Geometry: see drawing. Coordinates: mm, zero at the bounding-box minimum. Give positions to 0.01 mm unless a question says otherwise; leave off trailing zeros. Order: outer loops, then holes, each group sorted by start corner. A loop starts at its lowest first (then second) coordinate and runs counter-clockwise, first axis right, second up. Notation, with made-up numbers: (4.5, -35.5) -> (50.5, -35.5) arc R31 cw to (50.5, 1.5) -> close; hole circle Ø6 at (-11.75, 78). An arc over 180 degrees is marked (long way). Use one line per item in the form item = value. Start each with the question number.
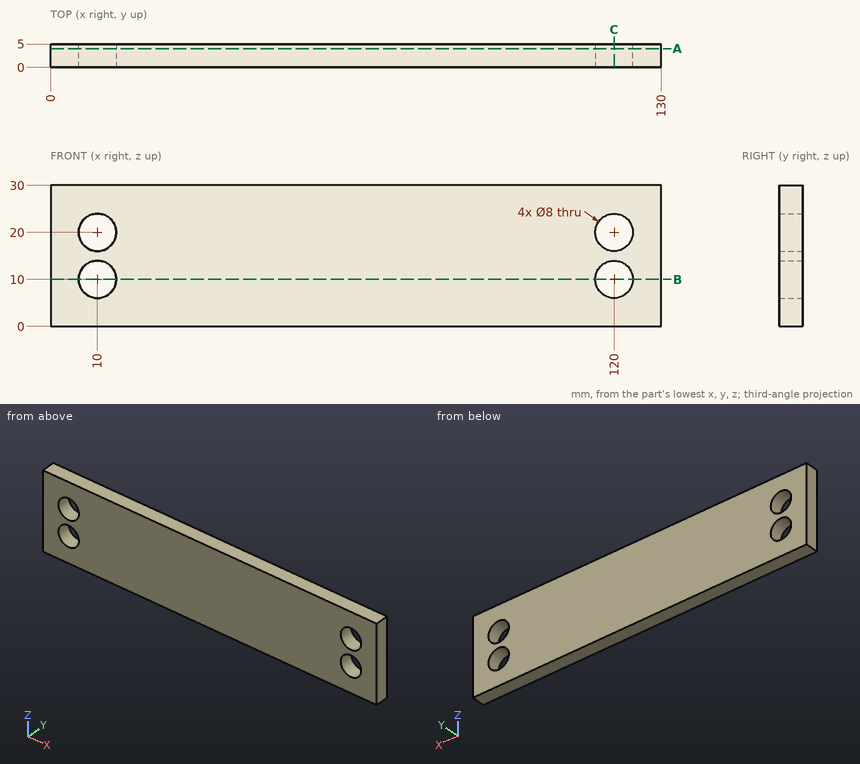
1) Material intervals for probe 1 along Z at (x, y) = (120, 1.6); probe 2 along X at (y, z) = (3.7, 9.75); probe 3 along X at (y, z) = (4.15, 10.75), sorted ascending.
2) Cut plane A-A, the plane y = 4. Return the cut outline in (x, z), plus the area to 3 significant figures.
3) Pin query (flat end, axial travel): pin 1 (7 mm diameter, centred on x = 10, z = 20, fed in from -Y). Return the tip coordinate at first contact, or that it passes through.
4) Cut plane C-C, the plane x = 120. Return the cut outline in (y, z).
5) Cut plane B-B, the plane z = 10. Return the cut outline in (x, y), plus the area to 3 significant figures.
Output values:
q1.probe_1 = 0 to 6, 14 to 16, 24 to 30
q1.probe_2 = 0 to 6.01, 13.99 to 116.01, 123.99 to 130
q1.probe_3 = 0 to 6.07, 13.93 to 116.07, 123.93 to 130
q2.outline = (0, 0) -> (130, 0) -> (130, 30) -> (0, 30) -> close; hole circle Ø8 at (10, 10); hole circle Ø8 at (10, 20); hole circle Ø8 at (120, 10); hole circle Ø8 at (120, 20)
q2.area = 3,700 mm^2
q3.pin_1 = through
q4.outline = (0, 0) -> (5, 0) -> (5, 6) -> (0, 6) -> close; (0, 14) -> (5, 14) -> (5, 16) -> (0, 16) -> close; (0, 24) -> (5, 24) -> (5, 30) -> (0, 30) -> close
q5.outline = (0, 0) -> (6, 0) -> (6, 5) -> (0, 5) -> close; (14, 0) -> (116, 0) -> (116, 5) -> (14, 5) -> close; (124, 0) -> (130, 0) -> (130, 5) -> (124, 5) -> close
q5.area = 570 mm^2
